Geometry: final body of the model. Coordinates: model frame, mm. Give positions to 0.01 mm unless a question says otherwise; leave off trailing zeros. Write each loop counter-clockwise with the first axis right and the second up, starting at its lowest first coordinate (ties: lowest second). Pieces come first, ordered by that corner, then holes. Notation, with made-up numbers: M 58,85 L 78,85 A25 cw 78,114 Z; hole C 31.5,-21.5 d7. An arc over 180 degrees is marked long. Use one line per item in the form item = value. Start each with the question number.
Item 1: Section query C-C on z = 16.5. Return loops of the section in (x, y) (3 decimals).
Item 2: Section query A-A on y = 75. Return loops of the section in (x, z) (3 decimals), then the cut area to 3 significant figures.
Item 3: Section query B-B on z = 23. Return loops of the section in (x, y) (3 decimals), then the cut area to 3 significant figures.
Item 4: Material intervals for line 1 along Y through (x, z) = (1.9, 25.4); line 2 along X through (y, z) = (60, 10.5) (3 decimals), sorted ascending. Write a range as from..to.
Item 5: Section query D-D on x = 46. Return loops of the section in (y, z) (3 decimals), then the cut area to 4 significant figures.
Item 6: Pull-direction query (Z, two-part tool) for faces 1 (the flat face through (26, 49, 0)), 2 (the cylindrical face through (1.565, 28.373, 23.25)), 3 (the flat face through (27, 49, 3.175)), 4 (the flat face through (3.175, 49, 27)); classes: released by +Z, released by -Z, zero draft, split by the parting line, or undercut.
Item 7: Contact query for flat-ended pins moving along their axis: P1, Ø13, axis at y = 75, z = 25.4, coming from the +X side (3 decimals); P2, Ø5, axis at x = 42, y = 69.5, coming from the +Z side (3 decimals); P3, Ø1.5, axis at x = 33, z = 5.5, coming from the -Y side. Output: stop coordinate, or through.
from build123d import *

# Parameters (mm, degrees)
BOSS_EXTRUDE1_DEPTH = 100
CUT_EXTRUDE1_REACH  = 125.131
SKETCH2_R           = 4


with BuildPart() as part:
    # Sketch1 → Boss-Extrude1 (new body)
    with BuildSketch(Plane(origin=(0, 0, 0), x_dir=(1, 0, 0), z_dir=(0, 1, 0))):
        Polygon((0, 0), (0, -50.8), (3.175, -50.8), (3.175, -3.175), (50.8, -3.175), (50.8, 0), align=None)
    extrude(amount=BOSS_EXTRUDE1_DEPTH)

    # Sketch2 → Cut-Extrude1 (cut, up to next)
    with BuildSketch(Plane(origin=(0, 0, 0), x_dir=(-1, 0, 0), z_dir=(0, 0, -1)), mode=Mode.PRIVATE) as cut_extrude1_sk1:
        with Locations((-25.4, 75)):
            Circle(SKETCH2_R)
    cut_extrude1_tool1 = extrude(cut_extrude1_sk1.sketch, amount=-CUT_EXTRUDE1_REACH, mode=Mode.PRIVATE) & part.part
    # Sketch2 → Cut-Extrude1 (cut, up to next)
    with BuildSketch(Plane(origin=(0, 0, 0), x_dir=(-1, 0, 0), z_dir=(0, 0, -1)), mode=Mode.PRIVATE) as cut_extrude1_sk2:
        with Locations((-25.4, 25)):
            Circle(SKETCH2_R)
    cut_extrude1_tool2 = extrude(cut_extrude1_sk2.sketch, amount=-CUT_EXTRUDE1_REACH, mode=Mode.PRIVATE) & part.part
    cut_extrude1_1 = cut_extrude1_tool1.solids().sort_by_distance((25.4, 75, 0))[0]
    add(cut_extrude1_1, mode=Mode.SUBTRACT)
    cut_extrude1_2 = cut_extrude1_tool2.solids().sort_by_distance((25.4, 25, 0))[0]
    add(cut_extrude1_2, mode=Mode.SUBTRACT)
    cut_extrude1 = cut_extrude1_1 + cut_extrude1_2  # Cut-Extrude1 as one shape, for the pattern or mirror that repeats it

    # Mirror1: Cut-Extrude1 across plane
    add(cut_extrude1.mirror(Plane(origin=(0, 0, 0), x_dir=(0.7071067811865478, 0, 0.7071067811865472), z_dir=(0.7071067811865475, 0, -0.7071067811865477))), mode=Mode.SUBTRACT)


solid = part.part
Answer sheet:
q1.outline = M 0,0 L 3.175,0 L 3.175,100 L 0,100 Z
q2.outline = M 0,0 L 21.4,0 L 21.4,3.175 L 3.175,3.175 L 3.175,21.4 L 0,21.4 Z; M 0,29.4 L 3.175,29.4 L 3.175,50.8 L 0,50.8 Z; M 29.4,0 L 50.8,0 L 50.8,3.175 L 29.4,3.175 Z
q2.area = 262 mm2
q3.outline = M 0,0 L 3.175,0 L 3.175,21.8 L 0,21.8 Z; M 0,28.2 L 3.175,28.2 L 3.175,71.8 L 0,71.8 Z; M 0,78.2 L 3.175,78.2 L 3.175,100 L 0,100 Z
q3.area = 277 mm2
q4.line_1 = 0..21, 29..71, 79..100
q4.line_2 = 0..3.175
q5.outline = M 0,0 L 100,0 L 100,3.175 L 0,3.175 Z
q5.area = 317.5 mm2
q6.face_1 = released by -Z
q6.face_2 = undercut
q6.face_3 = released by +Z
q6.face_4 = zero draft
q7.P1 = 3.175
q7.P2 = 3.175
q7.P3 = through
